Verification items for the finished model (mm, model axes). Face numbers are marked on the shaded views. A direction names the side the tool comes from. Round coordinates to 2 decimals unless told otherwise and drop trailing zeros. Write each loop counter-clockwise with the first axis right and the second up, starting at its lowest first coordinate (ties: lowest second). Pieces come first, ordered by that corner, then holes. Notation, with made-up numbers: (10.25, 89.5) - (58.25, 89.5) arc R12 cw to (58.25, 109.5) - close; hole circle Ø5 at (-21.75, 75.25). An arc over 180 degrees is marked (long way). Write each question's results on one line, items separated by ' | '.
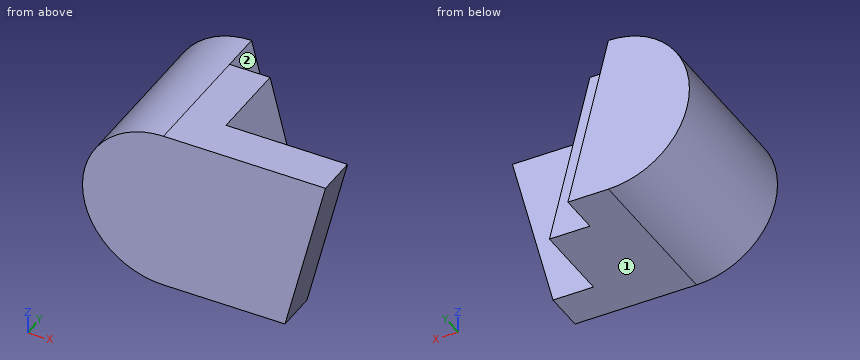
```python
from build123d import *

# Parameters (mm, degrees)
EXTRUDE_2_DEPTH = 4
EXTRUDE_3_DEPTH = 3
EXTRUDE_4_DEPTH = 1


with BuildPart() as part:
    # Sketch 1 → Extrude 2 (new body)
    with BuildSketch(Plane(origin=(0, 0, 0), x_dir=(1, 0, 0), z_dir=(0, 1, 0))):
        with BuildLine():
            Line((1, 2), (0, 2))
            ThreePointArc((0, 2), (-2, 0), (0, -2))
            Line((0, -2), (1, 2))
        make_face()
    extrude(amount=EXTRUDE_2_DEPTH)

    # Sketch 1_4 → Extrude 3 (add)
    with BuildSketch(Plane(origin=(0, 0, 0), x_dir=(1, 0, 0), z_dir=(0, 1, 0))):
        Polygon((2, 2), (1, 2), (0, -2), (1, -2), align=None)
    extrude(amount=EXTRUDE_3_DEPTH)

    # Sketch 1_5 → Extrude 4 (add)
    with BuildSketch(Plane(origin=(0, 0, 0), x_dir=(1, 0, 0), z_dir=(0, 1, 0))):
        with BuildLine():
            Line((0, 2), (3, 2))
            Line((3, 2), (4, -2))
            Line((4, -2), (0, -2))
            ThreePointArc((0, -2), (-2, 0), (0, 2))
        make_face()
    extrude(amount=EXTRUDE_4_DEPTH)


solid = part.part
```
(1) Section check A-A (z = 0). Record the cut outline in (x, y), plus the area to 3 significant figures.
Answer:
outline: (-2, 0) - (3.5, 0) - (3.5, 1) - (1.5, 1) - (1.5, 3) - (0.5, 3) - (0.5, 4) - (-2, 4) - close | area: 15.0 mm2
(2) Thickness scan on L1, parallel to Y at x = 2, z = 0.75; L2, parallel to Y at x = 1.3, z = -0.35; L3, parallel to X at y = 2.15, z = 0.9 (3 decimals). Record the ranges inside material, lowest first.
Answer:
L1: 0 to 1 | L2: 0 to 3 | L3: -1.786 to 1.275
(3) Section check D-D (x = 1.5). Record the cut outline in (y, z), plus the area to 3 significant figures.
Answer:
outline: (0, -2) - (3, -2) - (3, 0) - (1, 0) - (1, 2) - (0, 2) - close | area: 8.00 mm2
(4) Go/stop test with flat-tipped pins: pin 1 Ø1 at (y, z) = (0.5, 1) entering from +X (3 decimals); pin 2 Ø0.9 at (x, z) = (3, -0.5) entering from +Y; pin 3 Ø1 at (y, z) = (3, 1) entering from -X. Record where each tip stops, or that it passes through.
Answer:
pin 1: x = 3.875 | pin 2: y = 1 | pin 3: x = -1.94
(5) Section check C-C (y = 0.6). Record the cut outline in (x, z).
Answer:
outline: (0, -2) - (3, -2) - (4, 2) - (0, 2) arc R2 ccw to start
(6) Section check B-B (x = 0.1). Record the cut outline in (y, z).
Answer:
outline: (0, -2) - (4, -2) - (4, 1.6) - (3, 1.6) - (3, 2) - (0, 2) - close
(7) Set-up check for the marked faces 1 and 2: record each of +Z, -Z, +X, -X, +Y, -Y from which the full face is reachable in a straight line by a thin tool's end or side.
Answer:
face 1: -Z, +X, -X, +Y, -Y | face 2: +Z, +X, +Y
